Verification items for this drawing (mm, ordinates from the low corner). Coordinates: 2 decimals unless noted, no trailing zeros. Order: outer loops, then holes, each group sorted by start corner. A loop starts at its lowest first (then second) coordinate and runs counter-clockwise, first axis right, second up. Notation, with made-up numbers: M -22.75,-0.5 L 30.25,-0.5 A27 ccw 30.25,37.5 Z; hole C 15.25,23.5 d4. An arc over 180 degrees is marked long. Write item = value, one per line.
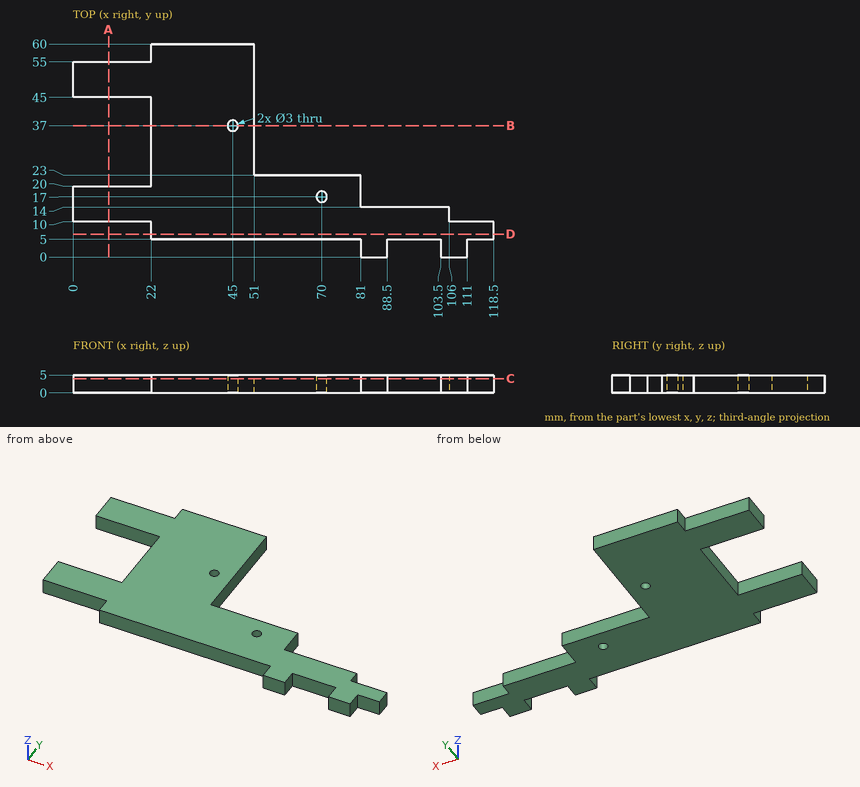
Item 1: Sectioned sample at C-C, the plane z = 4. Enter the section's corners in (x, y), then the cut area to 3 significant figures.
Report:
outline = M 0,10 L 22,10 L 22,5 L 81,5 L 81,0 L 88.5,0 L 88.5,5 L 103.5,5 L 103.5,0 L 111,0 L 111,5 L 118.5,5 L 118.5,10 L 106,10 L 106,14 L 81,14 L 81,23 L 51,23 L 51,60 L 22,60 L 22,55 L 0,55 L 0,45 L 22,45 L 22,20 L 0,20 Z; hole C 45,37 d3; hole C 70,17 d3
area = 2,920 mm^2
Item 2: Scan lines: L1, parallel to Y at x = 70, z = 2.1; L2, parallel to Y at x = 45, z = 2.2; L3, parallel to Y at x = 54, z = 0.7. Record each from-to range of solid material in increasing order. Write a range as from..to.
Report:
L1 = 5..15.5, 18.5..23
L2 = 5..35.5, 38.5..60
L3 = 5..23
Item 3: Sectioned sample at A-A, the plane x = 10. Enter the section's corners in (y, z), then the cut area to 3 significant figures.
Report:
outline = M 10,0 L 20,0 L 20,5 L 10,5 Z; M 45,0 L 55,0 L 55,5 L 45,5 Z
area = 100 mm^2
Item 4: Sectioned sample at B-B, the plane y = 37. Enter the section's corners in (x, z).
Report:
outline = M 22,0 L 43.5,0 L 43.5,5 L 22,5 Z; M 46.5,0 L 51,0 L 51,5 L 46.5,5 Z
Item 5: Gauge pin test, flat ends, axial feed: pin 1 (1.5 mm diameter, centred on y = 1.5, z = 2, fed in from +X); pin 2 (1.5 mm diameter, centred on x = 41.5, z = 2.5, fed in from -Y); pin 3 (1.5 mm diameter, centred on y = 15, z = 2.5, fed in from +X). Record the tip position at first contact, or that the pin passes through.
Report:
pin_1 = 111
pin_2 = 5
pin_3 = 81
Item 6: Sectioned sample at D-D, the plane y = 6.5. Enter the section's corners in (x, z).
Report:
outline = M 22,0 L 118.5,0 L 118.5,5 L 22,5 Z
